Build history of the part. All positions in model axes, mm. Face numbers are marked on the shaded views. A direction names the side the tool comes from. Give positions to 0.01 mm unless a question says otherwise; leave off trailing zeros. Order: outer loops, then holes, each group sorted by start corner. A loop starts at its lowest first (then second) coordinate and runs counter-clockwise, first axis right, second up. Notation, with made-up numbers: M 43,82 L 79,82 A21 ccw 79,93 Z; hole C 37.25,8.5 d3. An arc over 180 degrees is marked long. One line per item, written item: value.
from build123d import *

# Parameters (mm, degrees)
SKETCH1_R               = 2
BOSS_EXTRUDE1_DEPTH     = 5
SKETCH2_W               = 10
SKETCH2_H               = 20
BOSS_EXTRUDE2_DEPTH     = 9
SKETCH3_W               = 20
SKETCH3_H               = 4
BOSS_EXTRUDE3_DEPTH     = 4
SKETCH4_W               = 10
SKETCH4_H               = 13.5
BOSS_EXTRUDE4_DEPTH     = 2
CUT_EXTRUDE1_DEPTH      = 46.397604562
CUT_EXTRUDE1_DEPTH_BACK = 46.397604562
SKETCH5_R               = 1.27


with BuildPart() as part:
    # Sketch1 → Boss-Extrude1 (new body)
    with BuildSketch(Plane.XY):
        Polygon((16.807359313, 21.05), (11.05, 21.05), (11.05, -21.05), (16.807359313, -21.05), (21.05, -16.807359313), (21.05, 16.807359313), align=None)
        with Locations((15.5, -15.5)):
            Circle(SKETCH1_R, mode=Mode.SUBTRACT)
        with Locations((15.5, 15.5)):
            Circle(SKETCH1_R, mode=Mode.SUBTRACT)
    extrude(amount=BOSS_EXTRUDE1_DEPTH)

    # Sketch2 → Boss-Extrude2 (add)
    with BuildSketch(Plane.XY.offset(5)):
        with Locations((16.05, 0)):
            Rectangle(SKETCH2_W, SKETCH2_H)
    extrude(amount=BOSS_EXTRUDE2_DEPTH)

    # Sketch3 → Boss-Extrude3 (add)
    with BuildSketch(Plane.XY.offset(14)):
        with Locations((21.05, 4.75)):
            Rectangle(SKETCH3_W, SKETCH3_H)
        with Locations((21.05, -4.75)):
            Rectangle(SKETCH3_W, SKETCH3_H)
    extrude(amount=BOSS_EXTRUDE3_DEPTH)

    # Sketch4 → Boss-Extrude4 (add)
    with BuildSketch(Plane(origin=(0, 0, 14), x_dir=(-1, 0, 0), z_dir=(0, 0, -1))):
        with Locations((-26.05, 0)):
            Rectangle(SKETCH4_W, SKETCH4_H)
    extrude(amount=BOSS_EXTRUDE4_DEPTH)

    # Sketch5 → Cut-Extrude1 (cut, two sides: drawn at the far end of the back side and taken through both)
    with BuildSketch(Plane.XZ.offset(6.75).offset(-CUT_EXTRUDE1_DEPTH_BACK)):
        with Locations(Location((25.05, 15.27, 0), (0, 0, 270))):
            Circle(SKETCH5_R)
    extrude(amount=CUT_EXTRUDE1_DEPTH + CUT_EXTRUDE1_DEPTH_BACK, mode=Mode.SUBTRACT)


solid = part.part
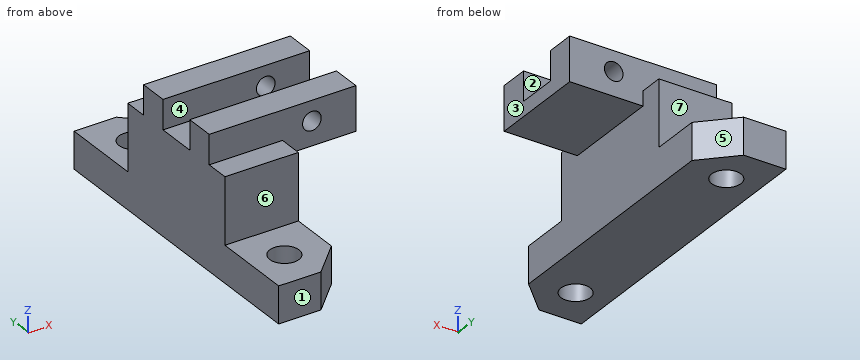
1) Saw through at A-A, the plane y = -15.5. Write the cut outline in (x, z), then the cut area to 3 significant figures.
Check values:
outline: M 11.05,0 L 13.5,0 L 13.5,5 L 11.05,5 Z; M 17.5,0 L 21.05,0 L 21.05,5 L 17.5,5 Z
area: 30.0 mm^2
2) Saw through at B-B, the plane x = 15.5. Write the cut outline in (y, z), then the cut area to 4 significant figures.
Check values:
outline: M -21.05,0 L -17.5,0 L -17.5,5 L -21.05,5 Z; M -13.5,0 L 13.5,0 L 13.5,5 L 10,5 L 10,14 L 6.75,14 L 6.75,18 L 2.75,18 L 2.75,14 L -2.75,14 L -2.75,18 L -6.75,18 L -6.75,14 L -10,14 L -10,5 L -13.5,5 Z; M 17.5,0 L 21.05,0 L 21.05,5 L 17.5,5 Z
area: 382.5 mm^2
3) Pin check, flat tips, straight feed: pin 1 (3 mm diameter, centred on x = 16.5, z = 16.5, fed in from -Y); pin 2 (4.5 mm diameter, centred on x = 14, z = 9, fed in from +Y); pin 3 (3.5 mm diameter, centred on x = 25.05, z = 15.27, fed in from +Y). Stop position of each tip, or through.
Check values:
pin 1: y = -6.75
pin 2: y = 10
pin 3: y = 6.75
4) Saw through at D-D, the plane z = 15.27. Write the cut outline in (x, y), then the cut area to 3 significant figures.
Check values:
outline: M 11.05,-6.75 L 23.78,-6.75 L 23.78,-2.75 L 11.05,-2.75 Z; M 11.05,2.75 L 23.78,2.75 L 23.78,6.75 L 11.05,6.75 Z; M 26.32,-6.75 L 31.05,-6.75 L 31.05,-2.75 L 26.32,-2.75 Z; M 26.32,2.75 L 31.05,2.75 L 31.05,6.75 L 26.32,6.75 Z
area: 140 mm^2
5) Mould opens along Y. For the marked faces 1, 2 and 3 say: released by +Y, released by -Y, zero draft, split by the parting line, or undercut.
Check values:
face 1: released by -Y
face 2: undercut
face 3: zero draft
6) Saw through at C-C, the plane z = 3.75. Write the cut outline in (x, y), then the cut area to 3 significant figures.
Check values:
outline: M 11.05,-21.05 L 16.81,-21.05 L 21.05,-16.81 L 21.05,16.81 L 16.81,21.05 L 11.05,21.05 Z; hole C 15.5,-15.5 d4; hole C 15.5,15.5 d4
area: 378 mm^2
7) Drill centre lines: probe 1 along Y at (x, z) = (15.5, 2.65); probe 2 along Z at (x, y) = (25.05, 4.8); probe 3 along Y at (x, z) = (30, 16.75). Where is each one in solid material? Low to high. Write a range as from..to.
Check values:
probe 1: -21.05..-17.5, -13.5..13.5, 17.5..21.05
probe 2: 12..14, 16.54..18
probe 3: -6.75..-2.75, 2.75..6.75
8) Tool access for the marked faces 4, 5, 6 and 7: list every direction of +Z, -Z, +X, -X, +Y, -Y with a clear straight run to the whole face (end or side of a thin tool).
Check values:
face 4: +Z, +X, -X
face 5: +Z, -Z, +X, +Y
face 6: +Z, +X, -X, -Y
face 7: +Z, +X, -X, +Y
